```python
from build123d import *

# Parameters (mm, degrees)
SKETCH_1_W                   = 40
SKETCH_1_H                   = 12
EXTRUDE_1_DEPTH              = 12
SKETCH_2_W                   = 9
SKETCH_2_H                   = 12
EXTRUDE_2_DEPTH              = 17
FILLET_1_R                   = 5
HOLE_WIZARD_M5_1_D           = 5.5
HOLE_WIZARD_M5_1_CBORE_D     = 10
HOLE_WIZARD_M5_1_CBORE_DEPTH = 5
CHAMFER_1_SIZE               = 0.5


with BuildPart() as part:
    # 草图1 → 凸台-拉伸1 (new body)
    with BuildSketch(Plane.XY):
        with Locations((20, 6)):
            Rectangle(SKETCH_1_W, SKETCH_1_H)
    extrude(amount=EXTRUDE_1_DEPTH)

    # 草图2 → 凸台-拉伸2 (add)
    with BuildSketch(Plane.XY.offset(12)):
        with Locations((4.5, 6)):
            Rectangle(SKETCH_2_W, SKETCH_2_H)
    extrude(amount=EXTRUDE_2_DEPTH)

    # 圆角1
    fillet_1_edges = [part.edges().sort_by_distance(p)[0] for p in [
        (9, 6, 12),
    ]]
    fillet(fillet_1_edges, radius=FILLET_1_R)

    # M5 六角凹头螺钉的柱形沉头孔1 (through all)
    with Locations(Plane.XY.offset(12)):
        with Locations((34, 6), (21, 6)):
            CounterBoreHole(HOLE_WIZARD_M5_1_D / 2, HOLE_WIZARD_M5_1_CBORE_D / 2, HOLE_WIZARD_M5_1_CBORE_DEPTH)

    # 倒角1
    chamfer_1_edges = [part.edges().sort_by_distance(p)[0] for p in [
        (40, 6, 12),
        (27, 12, 12),
        (9, 0, 23),
        (9, 12, 23),
        (0, 6, 29),
        (4.5, 0, 29),
        (9, 6, 29),
        (4.5, 12, 29),
        (27, 0, 12),
        (10.464466094, 12, 13.464466094),
        (10.464466094, 0, 13.464466094),
        (20, 12, 0),
        (40, 6, 0),
        (20, 0, 0),
        (0, 6, 0),
        (0, 12, 14.5),
        (40, 12, 6),
        (40, 0, 6),
        (0, 0, 14.5),
    ]]
    chamfer(chamfer_1_edges, length=CHAMFER_1_SIZE)


solid = part.part
```
Verification items for the finished model (mm, model axes). A direction names the side the tool comes from. Give positions to 0.01 mm unless a question says otherwise; leave off trailing zeros. Order: outer loops, then holes, each group sorted by start corner. A loop starts at its lowest first (then second) coordinate and runs counter-clockwise, first axis right, second up. Notation, with made-up numbers: (49, -20.75) -> (89, -20.75) arc R18 ccw to (89, -3.75) -> close; hole circle Ø8 at (4, 21). An arc over 180 degrees is marked (long way). Use a Markdown table: item, result.
1) Section check A-A, the plane y = 6. Record the boundary of the cut face in (x, z), then the cut area to 3 significant figures.
Results:
| item | result |
|---|---|
| outline | (0, 0.5) -> (0.5, 0) -> (18.25, 0) -> (18.25, 7) -> (16, 7) -> (16, 12) -> (14, 12) arc R5 cw to (9, 17) -> (9, 28.5) -> (8.5, 29) -> (0.5, 29) -> (0, 28.5) -> close; (23.75, 0) -> (31.25, 0) -> (31.25, 7) -> (29, 7) -> (29, 12) -> (26, 12) -> (26, 7) -> (23.75, 7) -> close; (36.75, 0) -> (39.5, 0) -> (40, 0.5) -> (40, 11.5) -> (39.5, 12) -> (39, 12) -> (39, 7) -> (36.75, 7) -> close |
| area | 461 mm² |
2) Section check C-C, the plane z = 18.75. Record the boundary of the cut face in (x, y), then the cut area to 4 significant figures.
Results:
| item | result |
|---|---|
| outline | (0, 0.5) -> (0.5, 0) -> (8.5, 0) -> (9, 0.5) -> (9, 11.5) -> (8.5, 12) -> (0.5, 12) -> (0, 11.5) -> close |
| area | 107.5 mm² |
3) Mould release check, pull along Y, two halves, no side actions. Record for faces 4 (the flat face through (23.2, 3.8, 7)), 5 (the flat face through (15, 12, 8)), 6 (the cylindrical face through (19.92, 1.12, 9.54)), 7 (the flat face through (20, 9, 0)): pulls with the +Y half, pulls with the -Y half, needs draft (parallel to the pull), parting line crosses it, or undercut.
Results:
| item | result |
|---|---|
| face 4 | undercut |
| face 5 | pulls with the +Y half |
| face 6 | undercut |
| face 7 | needs draft |
4) Material ranges on probe 1 along Y at (x, z) = (21, 5); probe 2 along X at (y, z) = (8.5, 6.5); probe 3 along Y at (x, z) = (21, 8.5), recorded low to high.
Results:
| item | result |
|---|---|
| probe 1 | 0 to 3.25, 8.75 to 12 |
| probe 2 | 0 to 19.85, 22.15 to 32.85, 35.15 to 40 |
| probe 3 | 0 to 1, 11 to 12 |
5) Section check B-B, the plane x = 34. Record the boundary of the cut face in (y, z).
Results:
| item | result |
|---|---|
| outline | (0, 0.5) -> (0.5, 0) -> (3.25, 0) -> (3.25, 7) -> (1, 7) -> (1, 12) -> (0.5, 12) -> (0, 11.5) -> close; (8.75, 0) -> (11.5, 0) -> (12, 0.5) -> (12, 11.5) -> (11.5, 12) -> (11, 12) -> (11, 7) -> (8.75, 7) -> close |
6) Section check D-D, the plane x = 27.5. Record the boundary of the cut face in (y, z).
Results:
| item | result |
|---|---|
| outline | (0, 0.5) -> (0.5, 0) -> (11.5, 0) -> (12, 0.5) -> (12, 11.5) -> (11.5, 12) -> (0.5, 12) -> (0, 11.5) -> close |
7) Depth check by flat-ended pin: pin 1 Ø6 at (x, y) = (21, 6) entering from +Z; pin 2 Ø3.5 at (x, y) = (21, 6) entering from +Z; pin 3 Ø5.5 at (y, z) = (7.5, 21.5) entering from +X. Enter the tip coordinate at first touch or a pass-through.
Results:
| item | result |
|---|---|
| pin 1 | z = 7 |
| pin 2 | through |
| pin 3 | x = 9 |
8) Tool access check on faces 1 (the flat face through (36.2, 3.8, 7)), 2 (the flat face through (9, 6, 23)), 3 (the cylindrical face through (36.747, 6.121, 3.451)). Record the directions out of +Z, -Z, +X, -X, +Y, -Y that give a thin tool (end or side, any length) a straight path to the whole face; none if there is none.
Results:
| item | result |
|---|---|
| face 1 | +Z |
| face 2 | +Z, +X, +Y, -Y |
| face 3 | +Z, -Z |
